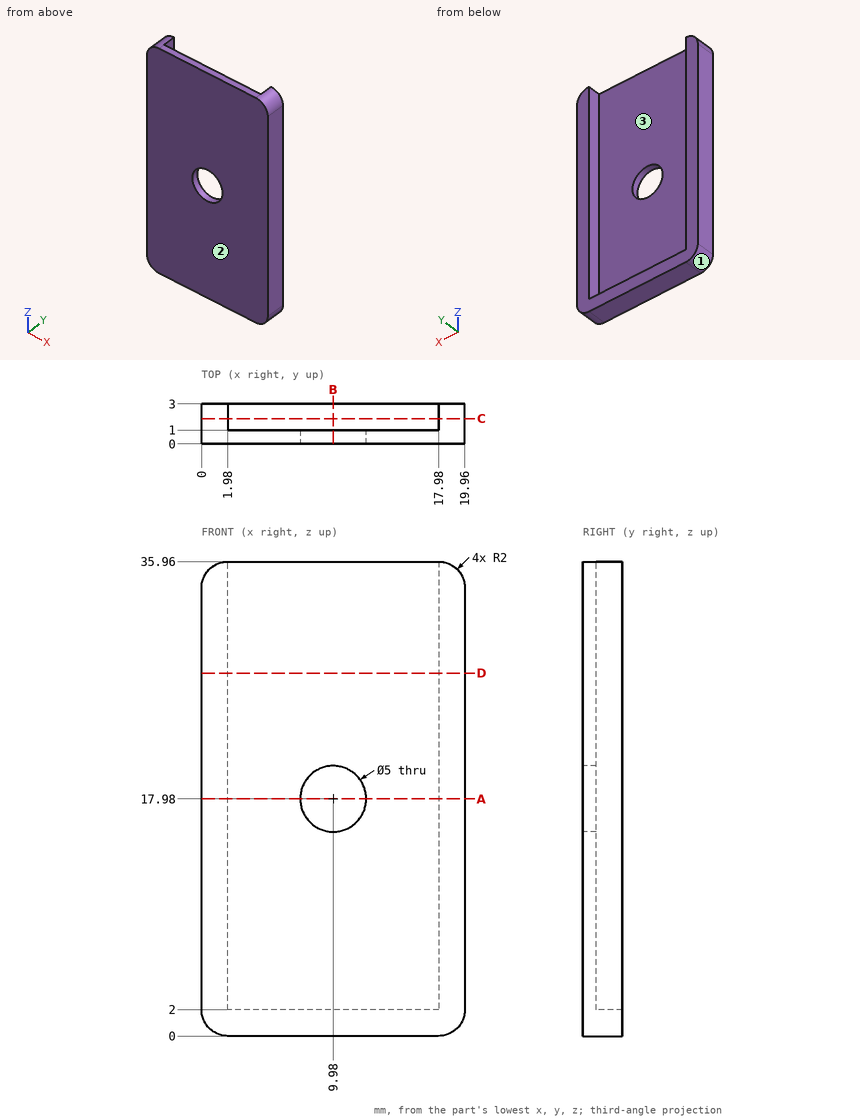
The figure shows three views and two pictorial views of one solid part (mm, origin at its lowest corner). Answer the questions. Give positions to 0.01 mm unless a question says otherwise; leave off trailing zeros. Write each loop counter-clockwise with the first axis right and the second up, starting at its lowest first coordinate (ties: lowest second). Pieces come first, ordered by that corner, then holes. Notation, with made-up numbers: (89.5, -23.5) - (96.5, -23.5) arc R35 cw to (96.5, 13.5) - close; hole circle Ø4 at (89, -28). An arc over 180 degrees is marked (long way). Return JSON: item names as keys, results as strings.
Q1. Given P1, Ø1.5, axis at x = 16.5, z = 13, coming from the +Y side; P2, Ø0.6, axis at x = 11, y = 2.5, coming from the +Z side; P3, Ø4, axis at x = 9.98, z = 17.98, coming from the -Y side, each flat-ended and moving along its own axis, determine where each tip first touches the part or whether it passes through.
Reply:
{"P1": "y = 1", "P2": "z = 2", "P3": "through"}
Q2. For a pull along X with two mould halves and no side action, classify the marked faces 1, 2 and 3 as released by +X, released by -X, zero draft, split by the parting line, or undercut.
Reply:
{"face 1": "released by -X", "face 2": "zero draft", "face 3": "undercut"}
Q3. A cutting plane is placed at D-D, the plane z = 27.5. Determine the outline of the cut face in (x, y).
Reply:
{"outline": "(0, 0) - (19.96, 0) - (19.96, 3) - (17.98, 3) - (17.98, 1) - (1.98, 1) - (1.98, 3) - (0, 3) - close"}
Q4. Consider line 1 along X through (y, z) = (2.4, 26.5); line 2 along Z through (x, y) = (9.98, 0.6); line 3 along Y through (x, z) = (7, 34). Determine where each line is inside the solid, lowest interval first. Write a range as [from, to].
Reply:
{"line 1": "[0, 1.98], [17.98, 19.96]", "line 2": "[0, 15.48], [20.48, 35.96]", "line 3": "[0, 1]"}
Q5. A cutting plane is placed at B-B, the plane x = 9.98. Determine the outline of the cut face in (y, z), and give its area (3 significant figures).
Reply:
{"outline": "(0, 0) - (3, 0) - (3, 2) - (1, 2) - (1, 15.48) - (0, 15.48) - close; (0, 20.48) - (1, 20.48) - (1, 35.96) - (0, 35.96) - close", "area": "35.0 mm²"}
Q6. A cutting plane is placed at C-C, the plane y = 1.9. Determine the outline of the cut face in (x, z), and give its area (3 significant figures).
Reply:
{"outline": "(0, 2) arc R2 ccw to (2, 0) - (17.96, 0) arc R2 ccw to (19.96, 2) - (19.96, 33.96) arc R2 ccw to (17.98, 35.96) - (17.98, 2) - (1.98, 2) - (1.98, 35.96) arc R2 ccw to (0, 33.96) - close", "area": "171 mm²"}
Q7. A cutting plane is placed at A-A, the plane z = 17.98. Determine the outline of the cut face in (x, y).
Reply:
{"outline": "(0, 0) - (7.48, 0) - (7.48, 1) - (1.98, 1) - (1.98, 3) - (0, 3) - close; (12.48, 0) - (19.96, 0) - (19.96, 3) - (17.98, 3) - (17.98, 1) - (12.48, 1) - close"}
